Autodesk Inventor part; units mm, degrees
ref_plane "Work Plane1" through (0, 0, 96.012) normal (0, 0, 1) x (1, 0, 0)
ref_plane "Work Plane2" through (0, 0, -96.012) normal (0, 0, -1) x (-1, 0, 0)
ref_plane "YZ Plane" through (0, 0, 0) normal (1, 0, 0) x (0, 1, 0)
sketch "Sketch1" plane through (0, 0, 0) normal (0, 0, 1) x (1, 0, 0)
  line L0 (-118.4529, 91.44) -> (86.7029, 91.44)
  line L1 (137.5029, 40.64) -> (137.5029, -91.44)
  line L2 (137.5029, -91.44) -> (10.5029, -91.44)
  line L3 (-137.5029, -30.1879) -> (-137.5029, 72.39)
  line L4 (-137.5029, 72.39) -> (-137.5029, -30.1879)
  line L5 (86.7029, 91.44) -> (137.5029, 40.64)
  line L6 (-118.4529, 91.44) -> (-137.5029, 72.39)
  line L7 (137.5029, -91.44) -> (10.5029, -91.44)
  line L8 (10.5029, -91.44) -> (-8.146196, -40.20203)
  line L9 (10.5029, -91.44) -> (65.029209, -91.44) construction
  line L10 (-8.146196, -40.20203) -> (-79.70483, -12.227388)
  line L11 (-79.70483, -12.227388) -> (-97.665343, -30.1879)
  line L12 (-97.665343, -30.1879) -> (-137.5029, -30.1879)
extrude "Extrusion1" add sketch "Sketch1" along normal mid plane 137.16
sketch "Sketch2" plane through (0, 0, -68.58) normal (0, 0, -1) x (-1, 0, 0)
  line L0 (-137.5029, 40.64) -> (-137.5029, -91.44)
  line L1 (-137.5029, -91.44) -> (-10.5029, -91.44)
  line L2 (-10.5029, -91.44) -> (8.146196, -40.20203)
  line L3 (8.146196, -40.20203) -> (79.70483, -12.227388)
  line L4 (79.70483, -12.227388) -> (97.665343, -30.1879)
  line L5 (97.665343, -30.1879) -> (137.5029, -30.1879)
  line L6 (137.5029, -30.1879) -> (137.5029, 72.39)
  line L7 (137.5029, 72.39) -> (118.4529, 91.44)
  line L8 (118.4529, 91.44) -> (-86.7029, 91.44)
  line L9 (-86.7029, 91.44) -> (-137.5029, 40.64)
  point P0 (0, 0)
sketch "Sketch3" plane through (0, 0, 68.58) normal (0, 0, 1) x (1, 0, 0)
  line L0 (137.5029, -91.44) -> (137.5029, 40.64)
  line L1 (137.5029, 40.64) -> (86.7029, 91.44)
  line L2 (86.7029, 91.44) -> (-118.4529, 91.44)
  line L3 (-118.4529, 91.44) -> (-137.5029, 72.39)
  line L4 (-137.5029, 72.39) -> (-137.5029, -30.1879)
  line L5 (-137.5029, -30.1879) -> (-97.665343, -30.1879)
  line L6 (-97.665343, -30.1879) -> (-79.70483, -12.227388)
  line L7 (-79.70483, -12.227388) -> (-8.146196, -40.20203)
  line L8 (-8.146196, -40.20203) -> (10.5029, -91.44)
  line L9 (10.5029, -91.44) -> (137.5029, -91.44)
  point P0 (0, 0)
ref_plane "Work Plane1" through (0, 0, 96.012) normal (0, 0, 1) x (1, 0, 0)
ref_plane "Work Plane2" through (0, 0, -96.012) normal (0, 0, -1) x (-1, 0, 0)
sketch "Sketch4" plane through (0, 0, 96.012) normal (0, 0, 1) x (1, 0, 0)
  line L0 (-126.464731, 65.844437) -> (-126.464731, -22.902911)
  line L1 (-126.464731, -22.902911) -> (-106.411156, -22.902911)
  line L2 (-106.411156, -22.902911) -> (-89.052252, -5.544007)
  line L3 (-106.411156, -22.902911) -> (-81.511939, 1.996306)
  line L4 (-81.511939, 1.996306) -> (0.53602, -30.665165)
  line L5 (0.53602, -30.665165) -> (19.270518, -79.10194)
  line L6 (19.270518, -79.10194) -> (124.736838, -79.10194)
  line L7 (124.736838, -79.10194) -> (124.736838, 33.064062)
  line L8 (124.736838, 33.064062) -> (79.026361, 78.774539)
  line L9 (79.026361, 78.774539) -> (-113.534629, 78.774539)
  line L10 (-113.534629, 78.774539) -> (-126.464731, 65.844437)
  point P0 (0, 0)
sketch "Sketch4 outline for Loft1" plane through (0, 0, 96.012) normal (0, 0, 1) x (1, 0, 0)
  line L0 (-113.534629, 78.774539) -> (-126.464731, 65.844437)
  line L1 (79.026361, 78.774539) -> (-113.534629, 78.774539)
  line L2 (124.736838, 33.064062) -> (79.026361, 78.774539)
  line L3 (124.736838, -79.10194) -> (124.736838, 33.064062)
  line L4 (19.270518, -79.10194) -> (124.736838, -79.10194)
  line L5 (0.53602, -30.665165) -> (19.270518, -79.10194)
  line L6 (-81.511939, 1.996306) -> (0.53602, -30.665165)
  line L7 (-106.411156, -22.902911) -> (-81.511939, 1.996306)
  line L8 (-126.464731, -22.902911) -> (-106.411156, -22.902911)
  line L9 (-126.464731, 65.844437) -> (-126.464731, -22.902911)
loft "Loft1" add profiles "Sketch4 outline for Loft1" section 2 edges at (137.5029, -25.4, 68.58) (112.1029, 66.04, 68.58) (-15.875, 91.44, 68.58) (-127.9779, 81.915, 68.58) (-137.5029, 21.10105, 68.58) (-117.584121, -30.1879, 68.58) (-88.685086, -21.207644, 68.58) (-43.925513, -26.214709, 68.58) (1.178352, -65.821015, 68.58) (74.0029, -91.44, 68.58)
sketch "Sketch5" plane through (-113.534629, 78.774539, 96.012) normal (0, 0, 1) x (1, 0, 0)
  line L0 (-12.930103, -12.930103) -> (-12.930103, -101.67745)
  line L1 (-12.930103, -101.67745) -> (7.123473, -101.67745)
  line L2 (7.123473, -101.67745) -> (32.02269, -76.778233)
  line L3 (32.02269, -76.778233) -> (114.070648, -109.439704)
  line L4 (114.070648, -109.439704) -> (132.805147, -157.876479)
  line L5 (132.805147, -157.876479) -> (238.271467, -157.876479)
  line L6 (238.271467, -157.876479) -> (238.271467, -45.710478)
  line L7 (238.271467, -45.710478) -> (192.560989, 0)
  line L8 (192.560989, 0) -> (0, 0)
  line L9 (0, 0) -> (-12.930103, -12.930103)
  point P0 (113.534629, -78.774539)
extrude "Extrusion2" add sketch "Sketch5" against normal blind 192.024
loft "Loft2" add section 1 edges at (-126.464731, 21.470763, -96.012) (-119.99968, 72.309488, -96.012) (-17.254134, 78.774539, -96.012) (101.881599, 55.9193, -96.012) (124.736838, -23.018939, -96.012) (72.003678, -79.10194, -96.012) (9.903269, -54.883552, -96.012) (-40.487959, -14.33443, -96.012) (-93.961547, -10.453303, -96.012) (-116.437944, -22.902911, -96.012) section 2 edges at (137.5029, -25.4, -68.58) (74.0029, -91.44, -68.58) (1.178352, -65.821015, -68.58) (-43.925513, -26.214709, -68.58) (-88.685086, -21.207644, -68.58) (-117.584121, -30.1879, -68.58) (-137.5029, 21.10105, -68.58) (-127.9779, 81.915, -68.58) (-15.875, 91.44, -68.58) (112.1029, 66.04, -68.58)
sketch "Sketch6" plane through (86.7029, 91.44, -68.58) normal (0.7071068, 0.7071068, 0) x (-0.7071068, 0.7071068, 0)
  line L0 (0, 0) -> (0, 137.16)
  line L1 (-71.842049, 0) -> (-71.842049, 137.16)
  line L2 (0, 137.16) -> (0, 91.44)
  line L3 (-71.842049, 0) -> (-71.842049, 45.72)
  line L4 (-71.842049, 45.72) -> (0, 45.72)
  line L5 (0, 45.72) -> (0, 91.44)
  line L6 (0, 91.44) -> (-71.842049, 91.44)
  line L7 (-71.842049, 91.44) -> (-71.842049, 45.72)
  point P0 (-3.349636, 68.58)
  dimension "d44" = 45.72
  dimension "d45" = 45.72
extrude "Extrusion3" add sketch "Sketch6" along normal blind 7.62
sketch "Sketch7" plane through (-118.4529, 91.44, 68.58) normal (0, 1, 0) x (1, 0, 0)
  line L0 (0, 137.16) -> (0, 0)
  line L1 (0, 137.16) -> (0, 91.44)
  line L2 (205.1558, 0) -> (205.1558, 45.72)
  line L3 (205.1558, 45.72) -> (78.1558, 45.72)
  line L4 (78.1558, 45.72) -> (78.1558, 91.44)
  line L5 (78.1558, 91.44) -> (205.1558, 91.44)
  line L6 (205.1558, 91.44) -> (205.1558, 45.72)
  point P0 (118.4529, 68.58)
  dimension "d48" = 45.72
  dimension "d49" = 127
extrude "Extrusion4" add sketch "Sketch7" along normal blind 7.62
sketch "Sketch8" plane through (137.5029, -91.44, 68.58) normal (1, 0, 0) x (0, 0, -1)
  line L0 (45.72, 132.08) -> (91.44, 132.08)
  line L1 (91.44, 132.08) -> (91.44, 30.48)
  line L2 (91.44, 30.48) -> (45.72, 30.48)
  line L3 (45.72, 30.48) -> (45.72, 132.08)
  point P0 (68.58, 91.44)
  dimension "d52" = 101.6
extrude "Extrusion5" add sketch "Sketch8" along normal blind 7.62
sketch "Sketch9" plane through (92.091054, 96.828154, -22.86) normal (-0.7071068, 0.7071068, 0) x (-0.7071068, -0.7071068, 0)
  line L0 (7.62, 0) -> (7.62, 45.72)
  line L1 (7.62, 45.72) -> (0, 45.72)
  line L2 (0, 0) -> (0, 45.72)
  line L3 (7.62, 0) -> (0, 0)
  point P0 (133.586053, 22.86)
sketch "Sketch10" plane through (142.891054, 46.028154, 22.86) normal (0, 0, 1) x (0.7071068, 0.7071068, 0)
  line L0 (-7.62, 0) -> (-7.62, 71.842049)
  line L1 (-7.62, 0) -> (0, 0)
  line L2 (0, 71.842049) -> (0, 0)
  line L3 (-7.62, 71.842049) -> (0, 71.842049)
  line L4 (-7.62, 71.842049) -> (-2.257751, 77.255983)
  line L5 (-7.62, 0) -> (-2.231846, -5.388154)
  line L6 (-7.62, 0) -> (0, 0) construction
  line L7 (-2.231846, -5.388154) -> (0, 0)
  line L8 (-2.257751, 77.255983) -> (0, 71.842049)
  line L9 (0, 71.842049) -> (0, 0)
  point P0 (-133.586053, 68.492413)
  dimension "d55" = 7.62
  dimension "d56" = 7.62
  dimension "d57" = 45
extrude "Extrusion6" add sketch "Sketch10" against normal blind 45.72
sketch "Sketch11" plane through (145.1229, -91.44, 68.58) normal (1, 0, 0) x (0, 0, -1)
  line L0 (45.72, 30.48) -> (91.44, 30.48)
  line L1 (91.44, 132.08) -> (45.72, 132.08)
  line L2 (68.58, 132.08) -> (68.58, 30.48) construction
  line L3 (55.88, 119.38) -> (55.88, 43.18)
  line L4 (81.28, 43.18) -> (81.28, 119.38)
  arc A0 (81.28, 119.38) -> (55.88, 119.38) centre (68.58, 119.38) ccw
  arc A1 (55.88, 43.18) -> (81.28, 43.18) centre (68.58, 43.18) ccw
  point P0 (68.58, 91.44)
  point P1 (68.58, 81.28)
  dimension "d60" = 25.4
extrude "Extrusion7" add sketch "Sketch11" along normal blind 2.54
properties part number "Head"
Could you check a few things on this model? Use its own coordinates, in mm. A direction names the side the tool comes from. Round coordinates to 2 decimals unless told otherwise and drop trailing zeros. Write each loop counter-clockwise with the first axis right and the second up, starting at its lowest first coordinate (ties: lowest second). Pieces come first, ordered by that corner, then holes. Notation, with made-up numbers: (20.25, 32) -> (50.25, 32) arc R7 ccw to (50.25, 45) -> close; hole circle Ø3 at (54, -19.75). An arc over 180 degrees is marked (long way). Use a Markdown table: item, result.
1. For pin 1 Ø6 at (x, z) = (91.5, -21.5) entering from +Y; pin 2 Ø3 at (x, z) = (-31.5, 48.5) entering from +Y; pin 3 Ø0.8 at (x, y) = (146, -22.5) entering from +Z, each with a flat end and sliding along its axis, tell me the tip position at first contact or that it passes through.
Answer key:
| item | result |
|---|---|
| pin 1 | stops at y = 98.31 |
| pin 2 | stops at y = 91.44 |
| pin 3 | stops at z = 12.7 |
2. Which directions (+Z, -Z, +X, -X, +Y, -Y) give clear straight access to the entire face, cutting with the end or side of a thin tool? Please do faces 5 (the face through (107, 72, 22.86)), 6 (the face through (-40.297, 95, 0)), 7 (the face through (141, -60.96, 0)).
Answer key:
| item | result |
|---|---|
| face 5 | +Z, +X, +Y |
| face 6 | +Z, -Z, -X, +Y |
| face 7 | +Z, -Z, +X, -Y |
3. If we section it at A-A (z = -29.5): List the corners of the cut face in (x, y) for me.
Answer key:
| item | result |
|---|---|
| outline | (-137.5, -30.19) -> (-97.67, -30.19) -> (-79.7, -12.23) -> (-8.15, -40.2) -> (10.5, -91.44) -> (137.5, -91.44) -> (137.5, 40.64) -> (86.7, 91.44) -> (-118.45, 91.44) -> (-137.5, 72.39) -> close |
4. We'd pull the mould along X, two halves only. Please class faces 1 (the face through (-17, 91.44, -31)), 2 (the face through (-88.56, -21.08, -0.96)), 3 (the face through (-43.425, -26.411, -0.96)), 4 (the face through (147.663, -9, 0)): +X half, -X half, draft (parallel to the pull), parting line (faces both ways), or undercut.
Answer key:
| item | result |
|---|---|
| face 1 | draft |
| face 2 | undercut |
| face 3 | undercut |
| face 4 | +X half |
5. Please list where these lines run through material, in increasing order: probe 1 along X at (y, z) = (12, -62); probe 2 along Y at (x, z) = (85.5, 52); probe 3 along X at (y, z) = (38.5, 10).
Answer key:
| item | result |
|---|---|
| probe 1 | x = -137.5 to 137.5 |
| probe 2 | y = -91.44 to 91.44 |
| probe 3 | x = -137.5 to 145.12 |
